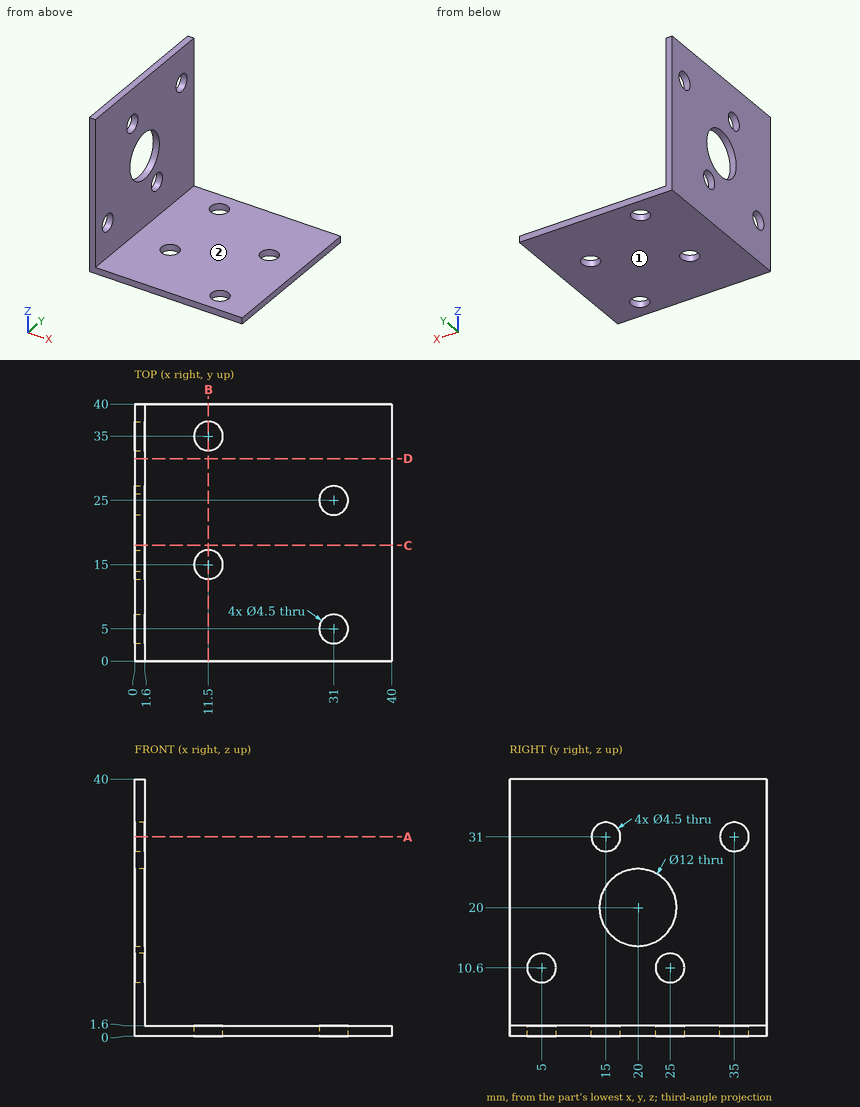
Input: dimensioned drawing with shaded views. Units: mm. Origin: part minimum x, y, z. A direction names the side the tool comes from. Give positions to 0.01 mm unless a question says otherwise; leave off trailing zeros. Loops run counter-clockwise (first coordinate to the right, second up) from the corner with the lowest first, then second, coordinate; pieces in that order, holes last. Notation, with made-up numbers: (-38, 52.5) -> (-15, 52.5) arc R15 cw to (-15, 64.5) -> close; hole circle Ø4 at (36.25, 60.25). An arc over 180 degrees is marked (long way). Return JSON: item names as keys, results as strings.
Item 1: Pin query (flat end, axial travel): P1, Ø14, axis at y = 20, z = 20, coming from the +X side; P2, Ø1.5, axis at y = 12, z = 30, coming from the -X side; P3, Ø6, axis at x = 31, y = 5, coming from the +Z side. Return the tip coordinate at first contact, or that it passes through.
Filled in:
{"P1": "x = 1.6", "P2": "x = 0", "P3": "z = 1.6"}
Item 2: Section C-C, the plane y = 18. Output: boundary loops of the cut face in (x, z), plus the area to 3 significant figures.
Filled in:
{"outline": "(0, 0) -> (40, 0) -> (40, 1.6) -> (1.6, 1.6) -> (1.6, 14.34) -> (0, 14.34) -> close; (0, 25.66) -> (1.6, 25.66) -> (1.6, 40) -> (0, 40) -> close", "area": "107 mm^2"}
Item 3: Section A-A, the plane z = 31. Output: boundary loops of the cut face in (x, y).
Filled in:
{"outline": "(0, 0) -> (1.6, 0) -> (1.6, 12.75) -> (0, 12.75) -> close; (0, 17.25) -> (1.6, 17.25) -> (1.6, 32.75) -> (0, 32.75) -> close; (0, 37.25) -> (1.6, 37.25) -> (1.6, 40) -> (0, 40) -> close"}
Item 4: Section B-B, the plane x = 11.5. Output: boundary loops of the cut face in (y, z).
Filled in:
{"outline": "(0, 0) -> (12.75, 0) -> (12.75, 1.6) -> (0, 1.6) -> close; (17.25, 0) -> (32.75, 0) -> (32.75, 1.6) -> (17.25, 1.6) -> close; (37.25, 0) -> (40, 0) -> (40, 1.6) -> (37.25, 1.6) -> close"}
Item 5: Section D-D, the plane y = 31.5. Output: boundary loops of the cut face in (x, z).
Filled in:
{"outline": "(0, 0) -> (40, 0) -> (40, 1.6) -> (1.6, 1.6) -> (1.6, 40) -> (0, 40) -> close"}
Item 6: Access query for the marked faces 1 and 2. Directions: +Z, -Z, +X, -X, +Y, -Y. A direction counts if a zero-diameter tool reaches every point of the face in a straight line with its end or side. Return the directions, or none.
Filled in:
{"face 1": "-Z, +X, -X, +Y, -Y", "face 2": "+Z, +X, +Y, -Y"}
Item 7: Line query: line 1 (Y direction, x = 31, z = 1); line 2 (Y direction, x = 1.05, z = 31); line 3 (Y direction, x = 0.65, z = 20). Output: solid intervals per line, ascending.
Filled in:
{"line 1": "0 to 2.75, 7.25 to 22.75, 27.25 to 40", "line 2": "0 to 12.75, 17.25 to 32.75, 37.25 to 40", "line 3": "0 to 14, 26 to 40"}
